Build history of the part. All positions in model axes, mm. Face numbers are marked on the shaded views. A direction names the side the tool comes from. Round coordinates to 2 decimals unless told otherwise and drop trailing zeros. Write each loop counter-clockwise with the first axis right and the second up, starting at its lowest first coordinate (ties: lowest second). Pieces come first, ordered by that corner, then holes.
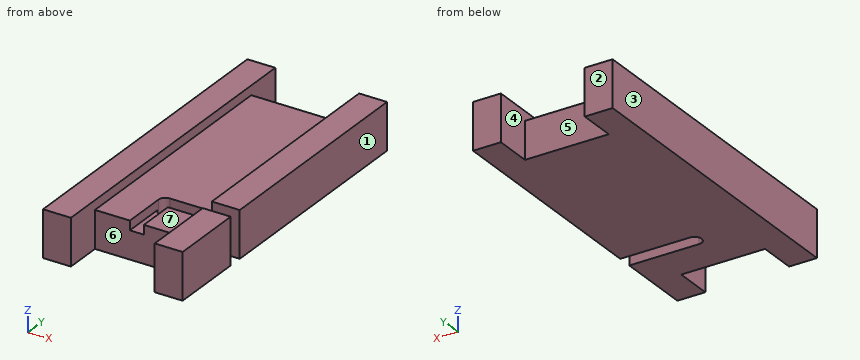
from build123d import *

# Parameters (mm, degrees)
F0_W     = 19.05
F0_H     = 33.02
F1_DEPTH = 6.35
F2_W     = 3.81
F2_H     = 6.35
F3_DEPTH = 5.08
F4_W     = 3.81
F4_H     = 6.35
F5_DEPTH = 5.08
F7_DEPTH = 2.54
F6_W     = 3.81
F6_H     = 1.905
F8_DEPTH = 6.35
F6_W_2   = 4.7625
F6_H_2   = 5.08
F9_DEPTH = 1.27


with BuildPart() as f1:
    # F0 (on Top) → F1 (new body)
    with BuildSketch(Plane.XY):
        Rectangle(F0_W, F0_H)
    extrude(amount=F1_DEPTH)

    # F2 (on face) → F3 (join)
    with BuildSketch(Plane.XZ.offset(16.51)):
        with Locations((-7.62, 3.175)):
            Rectangle(F2_W, F2_H)
        with Locations((7.62, 3.175)):
            Rectangle(F2_W, F2_H)
    extrude(amount=F3_DEPTH)

    # F4 (on face) → F5 (join)
    with BuildSketch(Plane(origin=(0, 16.51, 0), x_dir=(-1, 0, 0), z_dir=(0, 1, 0))):
        with Locations((-7.62, 3.175)):
            Rectangle(F4_W, F4_H)
        with Locations((7.62, 3.175)):
            Rectangle(F4_W, F4_H)
    extrude(amount=F5_DEPTH)

    # F6 (on face) → F7 (cut)
    with BuildSketch(Plane.XY.offset(6.35)):
        with BuildLine():
            Line((-0.9525, -16.51), (0.9525, -16.51))
            Line((0.9525, -16.51), (0.9525, -11.43))
            Line((0.9525, -11.43), (0, -11.43))
            ThreePointArc((0, -11.43), (-0.6735192091, -11.1510192091), (-0.9525, -10.4775))
            Line((-0.9525, -10.4775), (-0.9525, -16.51))
        make_face()
        with BuildLine():
            Line((0, -11.43), (0.9525, -11.43))
            Line((0.9525, -11.43), (0.9525, -10.4775))
            ThreePointArc((0.9525, -10.4775), (0.6735192091, -11.1510192091), (0, -11.43))
        make_face()
    extrude(amount=-F7_DEPTH, mode=Mode.SUBTRACT)

    # F6 (on face) → F8 (cut)
    with BuildSketch(Plane.XY.offset(6.35)):
        with BuildLine():
            Line((0, -10.4775), (0, -9.525))
            ThreePointArc((0, -9.525), (-0.6735192091, -9.8039807909), (-0.9525, -10.4775))
            Line((-0.9525, -10.4775), (0, -10.4775))
        make_face()
        with BuildLine():
            ThreePointArc((-0.9525, -10.4775), (-0.6735192091, -11.1510192091), (0, -11.43))
            Line((0, -11.43), (0, -10.4775))
            Line((0, -10.4775), (-0.9525, -10.4775))
        make_face()
        with BuildLine():
            ThreePointArc((0.9525, -10.4775), (0.6735192091, -9.8039807909), (0, -9.525))
            Line((0, -9.525), (0, -10.4775))
            Line((0, -10.4775), (0.9525, -10.4775))
        make_face()
        with BuildLine():
            Line((0, -10.4775), (0, -11.43))
            ThreePointArc((0, -11.43), (0.6735192091, -11.1510192091), (0.9525, -10.4775))
            Line((0.9525, -10.4775), (0, -10.4775))
        make_face()
        with BuildLine():
            Line((0.9525, -11.43), (5.715, -11.43))
            Line((5.715, -11.43), (5.715, -9.525))
            Line((5.715, -9.525), (0, -9.525))
            ThreePointArc((0, -9.525), (0.6735192091, -9.8039807909), (0.9525, -10.4775))
            Line((0.9525, -10.4775), (0.9525, -11.43))
        make_face()
        with Locations((7.62, -10.4775)):
            Rectangle(F6_W, F6_H)
        with BuildLine():
            Line((0, -11.43), (0.9525, -11.43))
            Line((0.9525, -11.43), (0.9525, -10.4775))
            ThreePointArc((0.9525, -10.4775), (0.6735192091, -11.1510192091), (0, -11.43))
        make_face()
    extrude(amount=-F8_DEPTH, mode=Mode.SUBTRACT)

    # F6 (on face) → F9 (cut)
    with BuildSketch(Plane.XY.offset(6.35)):
        with BuildLine():
            Line((0, -9.525), (5.715, -9.525))
            Line((5.715, -9.525), (5.715, 16.51))
            Line((5.715, 16.51), (-5.715, 16.51))
            Line((-5.715, 16.51), (-5.715, -16.51))
            Line((-5.715, -16.51), (-0.9525, -16.51))
            Line((-0.9525, -16.51), (-0.9525, -10.4775))
            ThreePointArc((-0.9525, -10.4775), (-0.6735192091, -9.8039807909), (0, -9.525))
        make_face()
        with Locations((3.33375, -13.97)):
            Rectangle(F6_W_2, F6_H_2)
    extrude(amount=-F9_DEPTH, mode=Mode.SUBTRACT)


solid = f1.part
1) Slice it at A-A (z = 5.5). Write the cut outline in (x, y) (3 decimals), plus the area to 3 significant figures.
Results:
outline: (-9.525, -21.59) - (-5.715, -21.59) - (-5.715, 21.59) - (-9.525, 21.59) - close; (5.715, -21.59) - (9.525, -21.59) - (9.525, -11.43) - (5.715, -11.43) - close; (5.715, -9.525) - (9.525, -9.525) - (9.525, 21.59) - (5.715, 21.59) - close
area: 322 mm2
2) Which spindle directions (+Z, -Z, +X, -X, +Y, -Y) get a long thin tool onto all of the face, cutting with end or side? Do the marked faces 5, 6 and 7. Say none if no direction does.
Results:
face 5: +Z, -Z, +Y
face 6: +Z, -Z, -Y
face 7: +Z, +Y, -Y
3) Wall check: L1, parallel to Y at x = 8.75, z = 5.5 (3 decimals); L2, parallel to Y at x = 1.5, z = 2 (3 decimals); L3, parallel to X at y = -2, z = 5.5 (3 decimals). Give the ranges that are in metal, low to high.
Results:
L1: y = -21.59 to -11.43, -9.525 to 21.59
L2: y = -16.51 to -11.43, -9.525 to 16.51
L3: x = -9.525 to -5.715, 5.715 to 9.525
4) Mould opens along X. For the marked faces 1, 2, 3 and 4 say: released by +X, released by -X, zero draft, split by the parting line, or undercut.
Results:
face 1: released by +X
face 2: zero draft
face 3: released by -X
face 4: undercut
5) Pin check, flat tips, straight feed: pin 1 Ø5 at (x, y) = (-4, -8) entering from +Z; pin 2 Ø1.5 at (x, z) = (-1, 2.5) entering from -Y; pin 3 Ø2 at (x, y) = (-4.5, 14) entering from +Z; pin 4 Ø1 at (x, y) = (0, -14.5) entering from +Z. Stop position of each tip, or through.
Results:
pin 1: stops at z = 6.35
pin 2: stops at y = -16.51
pin 3: stops at z = 5.08
pin 4: stops at z = 3.81
6) Slice it at B-B (x = 4.25). Write the cut outline in (y, z) (3 decimals).
Results:
outline: (-16.51, 0) - (-11.43, 0) - (-11.43, 5.08) - (-16.51, 5.08) - close; (-9.525, 0) - (16.51, 0) - (16.51, 5.08) - (-9.525, 5.08) - close
7) Slice it at D-D (z = 0.5). Write the cut outline in (x, y) (1 decimal), plus the area to 3 significant figures.
Results:
outline: (-9.5, -21.6) - (-5.7, -21.6) - (-5.7, -16.5) - (5.7, -16.5) - (5.7, -21.6) - (9.5, -21.6) - (9.5, -11.4) - (0, -11.4) arc R1 cw to (0, -9.5) - (9.5, -9.5) - (9.5, 21.6) - (5.7, 21.6) - (5.7, 16.5) - (-5.7, 16.5) - (-5.7, 21.6) - (-9.5, 21.6) - close
area: 687 mm2
8) Slice it at C-C (y = -4). Write the cut outline in (x, z) (3 decimals), plus the area to 3 significant figures.
Results:
outline: (-9.525, 0) - (9.525, 0) - (9.525, 6.35) - (5.715, 6.35) - (5.715, 5.08) - (-5.715, 5.08) - (-5.715, 6.35) - (-9.525, 6.35) - close
area: 106 mm2
